Here's how the part is built. I have some questions about the finished solid (model axes, mm). Face numbers are marked on the shaded views. A direction names the side the tool comes from. Round coordinates to 2 decimals unless told otherwise and drop trailing zeros. Loops run counter-clockwise (first coordinate to the right, second up) from the corner with the lowest first, then second, coordinate; pieces in that order, holes last. Notation, with made-up numbers: (87, -2.5) - (94, -2.5) arc R13 cw to (94, 14.5) - close; hole circle Ø9 at (2.5, -29.75). An arc over 180 degrees is marked (long way). Return JSON: item names as keys, results as strings. Group by question number.
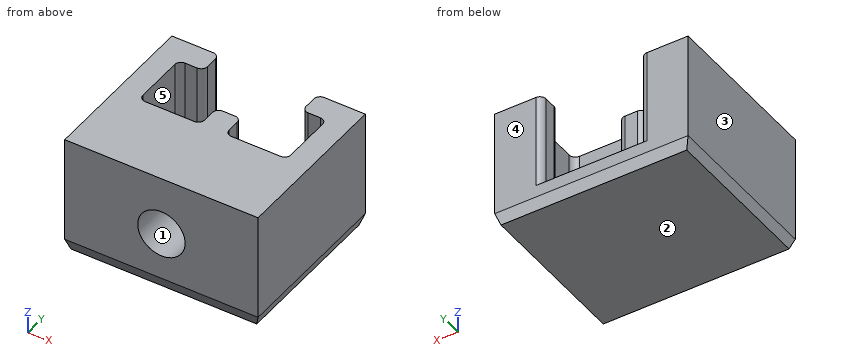
```python
from build123d import *

# Parameters (mm, degrees)
F1_DEPTH  = 10
F2_R      = 0.65
F4_DEPTH  = 2.5
F5_W      = 20.4
F5_H      = 6
F6_DEPTH  = 10
F7_DEPTH  = 2.5
F8_R      = 2.5
F9_DEPTH  = 7.5
F10_R     = 3
F10_R_2   = 2.5
F11_DEPTH = 1.5
F12_SIZE2 = 1.2
F12_SIZE  = 0.4


with BuildPart() as f1:
    # F0 (on Top) → F1 (new body)
    with BuildSketch(Plane.XY):
        Polygon((0, 11.5), (0, 0), (20.4, 0), (20.4, 11.5), (15.4, 11.5), (15.4, 8.9), (18, 8.9), (18, 2.4), (11.5, 2.4), (11.5, 5), (8.9, 5), (8.9, 2.4), (2.4, 2.4), (2.4, 8.9), (5, 8.9), (5, 11.5), align=None)
    extrude(amount=F1_DEPTH)

    # F2
    f2_edges = [f1.edges().sort_by_distance(p)[0] for p in [
        (2.4, 8.9, 5),
        (2.4, 2.4, 5),
        (11.5, 2.4, 5),
        (8.9, 2.4, 5),
        (18, 2.4, 5),
        (18, 8.9, 5),
        (15.4, 8.9, 5),
        (15.4, 11.5, 5),
        (5, 8.9, 5),
        (5, 11.5, 5),
        (11.5, 5, 5),
        (8.9, 5, 5),
    ]]
    fillet(f2_edges, radius=F2_R)

    # F3 (on face) → F4 (join)
    with BuildSketch(Plane(origin=(0, 0, 0), x_dir=(1, 0, 0), z_dir=(0, 0, -1))):
        with BuildLine():
            ThreePointArc((5, -10.85), (4.8096194078, -11.3096194078), (4.35, -11.5))
            Line((4.35, -11.5), (16.05, -11.5))
            ThreePointArc((16.05, -11.5), (15.5903805922, -11.3096194078), (15.4, -10.85))
            Line((15.4, -10.85), (15.4, -9.55))
            ThreePointArc((15.4, -9.55), (15.5903805922, -9.0903805922), (16.05, -8.9))
            Line((16.05, -8.9), (17.35, -8.9))
            ThreePointArc((17.35, -8.9), (17.8096194078, -8.7096194078), (18, -8.25))
            Line((18, -8.25), (18, -3.05))
            ThreePointArc((18, -3.05), (17.8096194078, -2.5903805922), (17.35, -2.4))
            Line((17.35, -2.4), (12.15, -2.4))
            ThreePointArc((12.15, -2.4), (11.6903805922, -2.5903805922), (11.5, -3.05))
            Line((11.5, -3.05), (11.5, -4.35))
            ThreePointArc((11.5, -4.35), (11.3096194078, -4.8096194078), (10.85, -5))
            Line((10.85, -5), (9.55, -5))
            ThreePointArc((9.55, -5), (9.0903805922, -4.8096194078), (8.9, -4.35))
            Line((8.9, -4.35), (8.9, -3.05))
            ThreePointArc((8.9, -3.05), (8.7096194078, -2.5903805922), (8.25, -2.4))
            Line((8.25, -2.4), (3.05, -2.4))
            ThreePointArc((3.05, -2.4), (2.5903805922, -2.5903805922), (2.4, -3.05))
            Line((2.4, -3.05), (2.4, -8.25))
            ThreePointArc((2.4, -8.25), (2.5903805922, -8.7096194078), (3.05, -8.9))
            Line((3.05, -8.9), (4.35, -8.9))
            ThreePointArc((4.35, -8.9), (4.8096194078, -9.0903805922), (5, -9.55))
            Line((5, -9.55), (5, -10.85))
        make_face()
        with BuildLine():
            Line((20.4, 0), (0, 0))
            Line((0, 0), (0, -11.5))
            Line((0, -11.5), (4.35, -11.5))
            ThreePointArc((4.35, -11.5), (4.8096194078, -11.3096194078), (5, -10.85))
            Line((5, -10.85), (5, -9.55))
            ThreePointArc((5, -9.55), (4.8096194078, -9.0903805922), (4.35, -8.9))
            Line((4.35, -8.9), (3.05, -8.9))
            ThreePointArc((3.05, -8.9), (2.5903805922, -8.7096194078), (2.4, -8.25))
            Line((2.4, -8.25), (2.4, -3.05))
            ThreePointArc((2.4, -3.05), (2.5903805922, -2.5903805922), (3.05, -2.4))
            Line((3.05, -2.4), (8.25, -2.4))
            ThreePointArc((8.25, -2.4), (8.7096194078, -2.5903805922), (8.9, -3.05))
            Line((8.9, -3.05), (8.9, -4.35))
            ThreePointArc((8.9, -4.35), (9.0903805922, -4.8096194078), (9.55, -5))
            Line((9.55, -5), (10.85, -5))
            ThreePointArc((10.85, -5), (11.3096194078, -4.8096194078), (11.5, -4.35))
            Line((11.5, -4.35), (11.5, -3.05))
            ThreePointArc((11.5, -3.05), (11.6903805922, -2.5903805922), (12.15, -2.4))
            Line((12.15, -2.4), (17.35, -2.4))
            ThreePointArc((17.35, -2.4), (17.8096194078, -2.5903805922), (18, -3.05))
            Line((18, -3.05), (18, -8.25))
            ThreePointArc((18, -8.25), (17.8096194078, -8.7096194078), (17.35, -8.9))
            Line((17.35, -8.9), (16.05, -8.9))
            ThreePointArc((16.05, -8.9), (15.5903805922, -9.0903805922), (15.4, -9.55))
            Line((15.4, -9.55), (15.4, -10.85))
            ThreePointArc((15.4, -10.85), (15.5903805922, -11.3096194078), (16.05, -11.5))
            Line((16.05, -11.5), (20.4, -11.5))
            Line((20.4, -11.5), (20.4, 0))
        make_face()
    extrude(amount=F4_DEPTH)

    # F5 (on Top) → F6 (join, through all)
    with BuildSketch(Plane.XY):
        with Locations((10.2, -3)):
            Rectangle(F5_W, F5_H)
    extrude(amount=F6_DEPTH)

    # F7 (add, through all): a face of the model
    f7_faces = [f1.faces().sort_by_distance(p)[0] for p in [
        (10.2, -3, 0),
    ]]
    extrude(f7_faces, amount=F7_DEPTH)

    # F8 (on face) → F9 (cut)
    with BuildSketch(Plane.XZ.offset(6)):
        with Locations((10.2, 3.75)):
            Circle(F8_R)
    extrude(amount=-F9_DEPTH, mode=Mode.SUBTRACT)

    # F10 (on face) → F11 (cut)
    with BuildSketch(Plane.XZ.offset(-1.5)):
        with Locations((10.2, 3.75)):
            Circle(F10_R)
        with Locations((10.2, 3.75)):
            Circle(F10_R_2, mode=Mode.SUBTRACT)
    extrude(amount=F11_DEPTH, mode=Mode.SUBTRACT)

    # F12
    f12_edges = [f1.edges().sort_by_distance(p)[0] for p in [
        (20.4, 2.75, -2.5),
        (10.2, -6, -2.5),
        (0, 2.75, -2.5),
        (10.2, 11.5, -2.5),
    ]]
    f12_side = f1.faces().sort_by_distance((10.2, 2.75, -2.5))[0]
    chamfer(f12_edges, length=F12_SIZE, length2=F12_SIZE2, reference=f12_side)


solid = f1.part
```
Q1. Will these pins go through, and if not, where does the flat tip stop? pin 1 Ø3 at (x, z) = (10.2, 3.75) entering from -Y; pin 2 Ø0.6 at (x, z) = (10, 5.5) entering from +Y; pin 3 Ø2.5 at (x, z) = (7, 4) entering from +Y.
Q2. Imagine slicing it at D-D, the plane y = 7.75. List the corners of the cut face in (x, z) for me, and give its area (3 significant figures).
Q3. If we mould it in two halves opening along Y, with no side actions, what happens to the marked faces 3, 4 and 5? For each: +Y half, -Y half, draft (parallel to the pull), parting line (faces both ways), or undercut.
Q4. Imagine slicing it at B-B, the plane y = -2.75. List the corners of the cut face in (x, z) for me, and give its area (3 significant figures).
Q5. Imagine slicing it at A-A, the plane x = 10.2. List the corners of the cut face in (y, z) for me.
Q6. Please list where these lines run through material, in increasing order: line 1 (X direction, y = 3, z = 9); line 2 (Y direction, x = 3.25, z = 6); line 3 (Z direction, x = 10.2, y = -3.55).
Q7. For the marked faces 1 and 2, which set-ups out of +Z, -Z, +X, -X, +Y, -Y let a thin tool reach every point of the face, with its end or its side?
Output values:
{
 "1": {"pin 1": "stops at y = 1.5", "pin 2": "stops at y = 5", "pin 3": "stops at y = 2.4"},
 "2": {"outline": "(0, -1.3) - (0.4, -2.5) - (20, -2.5) - (20.4, -1.3) - (20.4, 10) - (18, 10) - (18, 0) - (2.4, 0) - (2.4, 10) - (0, 10) - close", "area": "98.5 mm^2"},
 "3": {"face 3": "draft", "face 4": "+Y half", "face 5": "undercut"},
 "4": {"outline": "(0, -1.3) - (0.4, -2.5) - (20, -2.5) - (20.4, -1.3) - (20.4, 10) - (0, 10) - close; hole circle Ø5 at (10.2, 3.75)", "area": "235 mm^2"},
 "5": {"outline": "(-6, -1.3) - (-5.6, -2.5) - (11.1, -2.5) - (11.5, -1.3) - (11.5, 0) - (5, 0) - (5, 10) - (-6, 10) - (-6, 6.25) - (0, 6.25) - (0, 6.75) - (1.5, 6.75) - (1.5, 0.75) - (0, 0.75) - (0, 1.25) - (-6, 1.25) - close"},
 "6": {"line 1": "x = 0 to 2.4, 8.9 to 11.5, 18 to 20.4", "line 2": "y = -6 to 2.4, 8.9 to 11.5", "line 3": "z = -2.5 to 1.25, 6.25 to 10"},
 "7": {"face 1": "-Y", "face 2": "-Z, +X, -X, +Y, -Y"}
}
